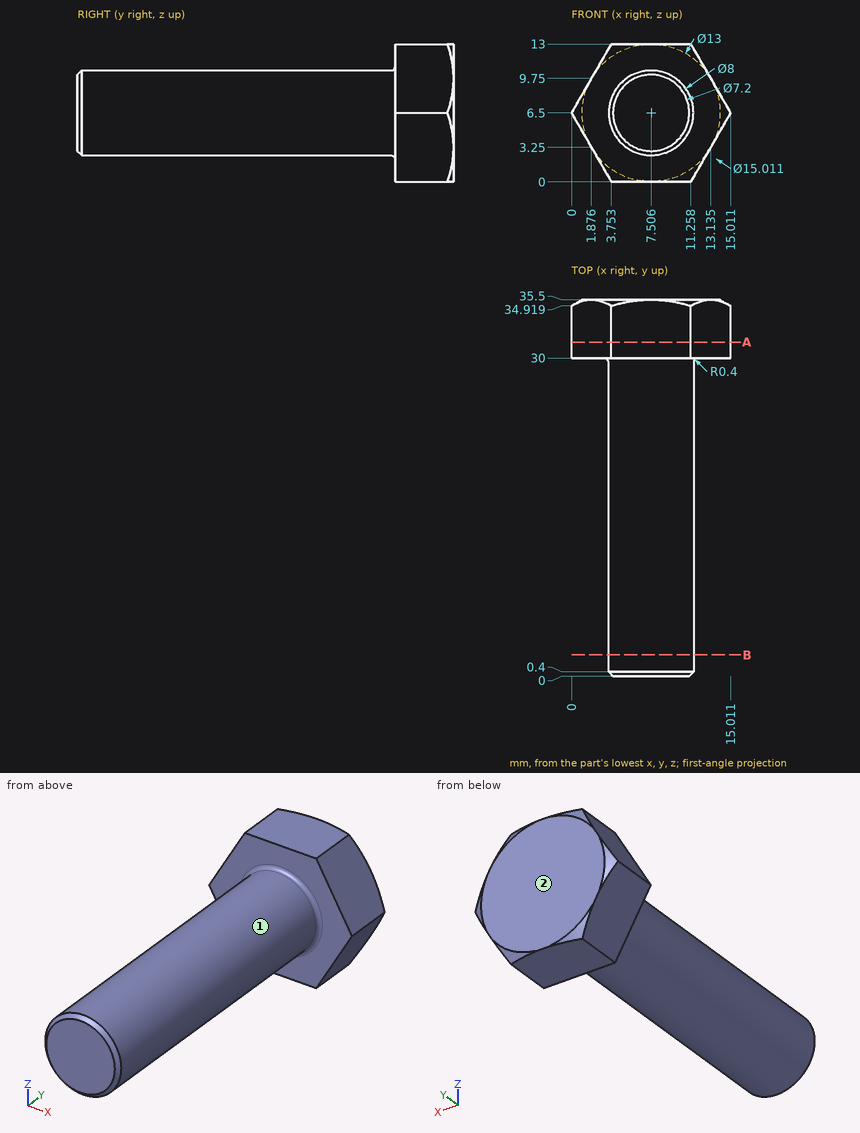
Print and shaded views of the part. All mm, measured from the part's lowest x, y and z. A direction names the side the tool comes from. Round coordinates to 2 decimals unless told otherwise and drop trailing zeros. Order: outer loops, then holes, each group sorted by start corner. A loop starts at its lowest first (then second) coordinate and runs counter-clockwise, first axis right, second up.
Q1. Wall check: L1, parallel to Z at x = 7.5, y = 7; L2, parallel to Y at x = 1.5, z = 5.25; L3, parallel to X at y = 9.5, z = 8.5. Give the ranges that are in metal, low to high.
Q2. Slice it at B-B (y = 2). Write the cut outline in (x, z) (1 decimal).
Q3. Drop flat-ended pins along their axis: pin 1 (3 mm diameter, centred on x = 9.5, y = 30.5, fed in from -Z); pin 2 (2 mm diameter, centred on x = 11, y = 27, fed in from +Z); pin 3 (1.5 mm diameter, centred on x = 8.5, y = 4.5, fed in from -Z); pin 4 (4 mm diameter, centred on y = 9, z = 11.5, fed in from +X). Give the stop position or say it passes through.
Q4. Slice it at A-A (y = 31.5). Write the cut outline in (x, z), and give its area (3 significant figures).
Q5. Which spindle directions (+Z, -Z, +X, -X, +Y, -Y) get a long thin tool onto all of the face, cutting with end or side? Do the marked faces 1 and 2. Say none if no direction does.
Results below:
1. L1: z = 2.5 to 10.5
1. L2: y = 30 to 35.5
1. L3: x = 4.04 to 10.97
2. outline: circle Ø8 at (7.5, 6.5)
3. pin 1: stops at z = 0
3. pin 2: stops at z = 9.63
3. pin 3: stops at z = 2.51
3. pin 4: stops at x = 10.15
4. outline: (0, 6.5) - (3.75, 0) - (11.26, 0) - (15.01, 6.5) - (11.26, 13) - (3.75, 13) - close
4. area: 146 mm2
5. face 1: -Y
5. face 2: +Z, -Z, +X, -X, +Y
